Verification items for the finished model (mm, model axes). Round coordinates to 2 decimals unless told otherwise and drop trailing zeros. Write each loop counter-clockwise with the first axis right and the second up, starting at its lowest first coordinate (ties: lowest second). Pieces come first, ordered by that corner, then holes. Notation, with made-up numbers: (-34.5, 36) -> (1.5, 36) arc R28 cw to (1.5, 59) -> close; hole circle Ø7 at (-10, 2). An arc over 180 degrees is marked (long way). Use CSV: the item, a comma, the result in double quotes.
Autodesk Fusion 360 part; units mm, degrees
sketch "Base" plane through (0, 0, 0) normal (0, 0, 1) x (1, 0, 0)
  line L0 (0, 0) -> (0, 31.75)
  line L1 (222.25, 0) -> (0, 0)
  line L2 (222.25, 31.75) -> (222.25, 0)
  line L3 (0, 31.75) -> (222.25, 31.75)
  line L4 (76.2, 12.7001) -> (25.4, 12.7001)
  line L5 (25.4, 19.05) -> (76.2, 19.05)
  line L6 (76.2, 19.05) -> (76.2, 12.7001)
  line L7 (25.4, 12.7001) -> (25.4, 19.05)
  line L8 (196.85, 19.05) -> (196.85, 12.7001)
  line L9 (146.05, 19.05) -> (196.85, 19.05)
  line L10 (146.05, 12.7001) -> (146.05, 19.05)
  line L11 (196.85, 12.7001) -> (146.05, 12.7001)
extrude "Extrude1" add sketch "Base" along normal blind 6.35
fillet "Fillet1" radius 6.35 1 edges at (222.25, 0, 3.175)
fillet "Fillet2" radius 6.35 1 edges at (222.25, 31.75, 3.175)
fillet "Fillet3" radius 6.35 1 edges at (0, 31.75, 3.175)
fillet "Fillet4" radius 6.35 1 edges at (0, 0, 3.175)
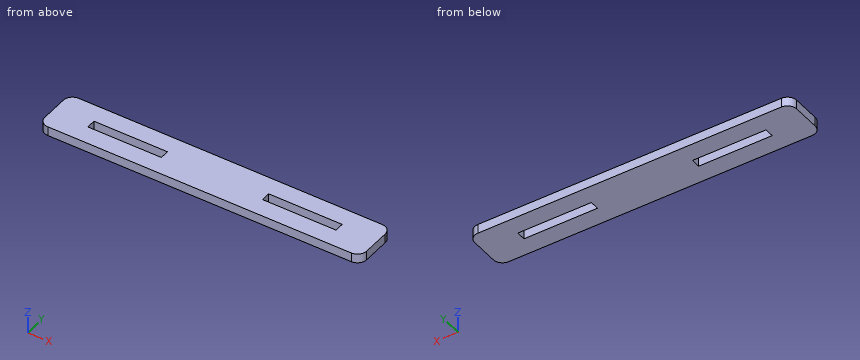
Q1. Go/stop test with flat-tipped pins: P1, Ø3, axis at y = 27.5, z = 2, coming from the +X side; P2, Ø3, axis at x = 46, z = 4, coming from the -Y side. Record where each tip stops, or that it passes through.
Filled in:
P1,"x = 222.22"
P2,"y = 0"
Q2. Section check B-B (y = 15). Record the cut outline in (x, z).
Filled in:
outline,"(0, 0) -> (25.4, 0) -> (25.4, 6.35) -> (0, 6.35) -> close; (76.2, 0) -> (146.05, 0) -> (146.05, 6.35) -> (76.2, 6.35) -> close; (196.85, 0) -> (222.25, 0) -> (222.25, 6.35) -> (196.85, 6.35) -> close"
Q3. Section check A-A (x = 50). Record the cut outline in (y, z), plus the area to 3 significant figures.
Filled in:
outline,"(0, 0) -> (12.7, 0) -> (12.7, 6.35) -> (0, 6.35) -> close; (19.05, 0) -> (31.75, 0) -> (31.75, 6.35) -> (19.05, 6.35) -> close"
area,"161 mm²"
Q4. Section check C-C (z = 1). Record the cut outline in (x, y), plus the area to 3 significant figures.
Filled in:
outline,"(0, 6.35) arc R6.35 ccw to (6.35, 0) -> (215.9, 0) arc R6.35 ccw to (222.25, 6.35) -> (222.25, 25.4) arc R6.35 ccw to (215.9, 31.75) -> (6.35, 31.75) arc R6.35 ccw to (0, 25.4) -> close; hole (25.4, 12.7) -> (76.2, 12.7) -> (76.2, 19.05) -> (25.4, 19.05) -> close; hole (146.05, 12.7) -> (196.85, 12.7) -> (196.85, 19.05) -> (146.05, 19.05) -> close"
area,"6,380 mm²"
Q5. Material ranges on L1, parallel to X at y = 19, z = 5.75; L2, parallel to Y at x = 152, z = 5.5; L3, parallel to X at y = 25.5, z = 1, recorded low to high.
Filled in:
L1,"0 to 25.4, 76.2 to 146.05, 196.85 to 222.25"
L2,"0 to 12.7, 19.05 to 31.75"
L3,"0 to 222.25"
